For this review, take the finished solid that the model builds, in its own axes (mm). Face numbers are marked on the shaded views. Coordinates: 2 decimals unless noted, no trailing zeros. Write each loop counter-clockwise with the first axis right and the second up, starting at its lowest first coordinate (ties: lowest second). Pieces come first, ordered by that corner, then holes. Notation, with made-up numbers: M -20.5,14.25 L 18.5,14.25 A33 ccw 18.5,53.25 Z; hole C -2,-17 d2. An arc over 180 degrees is marked long. Return JSON: item names as keys, results as strings.
Autodesk Inventor part; units mm, degrees
ref_plane "YZ Plane" through (0, 0, 0) normal (1, 0, 0) x (0, 1, 0)
ref_plane "XZ Plane" through (0, 0, 0) normal (0, 1, 0) x (-1, 0, 0)
ref_plane "XY Plane" through (0, 0, 0) normal (0, 0, 1) x (1, 0, 0)
sketch "0" plane through (0, 0, 0) normal (0, 0, 1) x (1, 0, 0)
  line L0 (4, 55.5) -> (4, 61.5)
  line L1 (4, 61.5) -> (14, 61.5)
  line L2 (14, 61.5) -> (14, 55.5)
  line L3 (20, 55.5) -> (18.5, 55.5)
  line L4 (18.5, 55.5) -> (18.5, 49.25)
  line L5 (18.5, 40.5) -> (15.5, 40.5)
  line L6 (15.5, 40.5) -> (15.5, 46.75)
  line L7 (14.25, 49.25) -> (15.5, 49.25)
  line L8 (19.75, 49.25) -> (19.75, 46.75)
  line L9 (19.75, 46.75) -> (18.5, 46.75)
  line L10 (14.25, 46.75) -> (14.25, 49.25)
  line L11 (15.5, 49.25) -> (15.5, 55.5)
  line L12 (15.5, 46.75) -> (14.25, 46.75)
  line L13 (18.5, 49.25) -> (19.75, 49.25)
  line L14 (15.5, 55.5) -> (14, 55.5)
  line L15 (20, 61.5) -> (30, 61.5)
  line L16 (20, 55.5) -> (20, 61.5)
  line L17 (18.5, 46.75) -> (18.5, 40.5)
  line L18 (-30, 61.5) -> (-20, 61.5)
  line L19 (-20, 61.5) -> (-20, 55.5)
  line L20 (-14, 55.5) -> (-15.5, 55.5)
  line L21 (-15.5, 55.5) -> (-15.5, 49.25)
  line L22 (-15.5, 40.5) -> (-18.5, 40.5)
  line L23 (-18.5, 40.5) -> (-18.5, 46.75)
  line L24 (-19.75, 49.25) -> (-18.5, 49.25)
  line L25 (-14.25, 49.25) -> (-14.25, 46.75)
  line L26 (-14.25, 46.75) -> (-15.5, 46.75)
  line L27 (-19.75, 46.75) -> (-19.75, 49.25)
  line L28 (-18.5, 49.25) -> (-18.5, 55.5)
  line L29 (-18.5, 46.75) -> (-19.75, 46.75)
  line L30 (-15.5, 49.25) -> (-14.25, 49.25)
  line L31 (-18.5, 55.5) -> (-20, 55.5)
  line L32 (-14, 61.5) -> (-4, 61.5)
  line L33 (-14, 55.5) -> (-14, 61.5)
  line L34 (-4, 61.5) -> (-4, 55.5)
  line L35 (-15.5, 46.75) -> (-15.5, 40.5)
  line L36 (-3, 55.5) -> (-4, 55.5)
  line L37 (3, 55.5) -> (4, 55.5)
  line L38 (30, 61.5) -> (30, 55.5)
  circle A0 centre (0, 0) radius 18
  line L39 (30, 55.5) -> (30, -4)
  line L40 (-30, -4) -> (-30, 61.5)
  arc A1 (-30, -4) -> (30, -4) centre (0, 8.5) ccw
  line L41 (-3, 19.5) -> (-3, 29.5)
  line L42 (-3, 29.5) -> (3, 29.5)
  line L43 (3, 29.5) -> (3, 19.5)
  line L44 (3, 19.5) -> (-3, 19.5)
  line L45 (-3, 35.5) -> (-3, 45.5)
  line L46 (3, 45.5) -> (3, 35.5)
  line L47 (3, 35.5) -> (-3, 35.5)
  circle A2 centre (0, 32.5) radius 1.6
  line L48 (-3, 45.5) -> (3, 45.5)
  line L49 (-3, 55.5) -> (3, 55.5)
  point P0 (-30, -4)
  point P1 (30, -4)
sketch "Эскиз3" plane through (0, 0, 0) normal (0, 0, 1) x (1, 0, 0)
  circle A0 centre (0, 0) radius 18
  circle A1 centre (0, 32.5) radius 1.6
  line L0 (30, 55.5) -> (30, -4)
  line L1 (-30, -4) -> (-30, 61.5)
  line L2 (-30, 61.5) -> (-20, 61.5)
  line L3 (30, 61.5) -> (30, 55.5)
  line L4 (20, 61.5) -> (30, 61.5)
  line L5 (20, 55.5) -> (20, 61.5)
  line L6 (20, 55.5) -> (18.5, 55.5)
  line L7 (18.5, 55.5) -> (18.5, 49.25)
  line L8 (18.5, 49.25) -> (19.75, 49.25)
  line L9 (19.75, 49.25) -> (19.75, 46.75)
  line L10 (19.75, 46.75) -> (18.5, 46.75)
  line L11 (18.5, 46.75) -> (18.5, 40.5)
  line L12 (18.5, 40.5) -> (15.5, 40.5)
  line L13 (15.5, 40.5) -> (15.5, 46.75)
  line L14 (15.5, 46.75) -> (14.25, 46.75)
  line L15 (14.25, 46.75) -> (14.25, 49.25)
  line L16 (14.25, 49.25) -> (15.5, 49.25)
  line L17 (15.5, 49.25) -> (15.5, 55.5)
  line L18 (15.5, 55.5) -> (14, 55.5)
  line L19 (4, 61.5) -> (14, 61.5)
  line L20 (4, 55.5) -> (4, 61.5)
  line L21 (-3, 55.5) -> (3, 55.5)
  line L22 (3, 55.5) -> (4, 55.5)
  line L23 (14, 61.5) -> (14, 55.5)
  line L24 (-14, 61.5) -> (-4, 61.5)
  line L25 (-4, 61.5) -> (-4, 55.5)
  line L26 (-14, 55.5) -> (-15.5, 55.5)
  line L27 (-15.5, 55.5) -> (-15.5, 49.25)
  line L28 (-18.5, 49.25) -> (-18.5, 55.5)
  line L29 (-18.5, 55.5) -> (-20, 55.5)
  line L30 (-20, 61.5) -> (-20, 55.5)
  line L31 (-19.75, 49.25) -> (-18.5, 49.25)
  line L32 (-19.75, 46.75) -> (-19.75, 49.25)
  line L33 (-18.5, 46.75) -> (-19.75, 46.75)
  line L34 (-18.5, 40.5) -> (-18.5, 46.75)
  line L35 (-15.5, 40.5) -> (-18.5, 40.5)
  line L36 (-15.5, 46.75) -> (-15.5, 40.5)
  line L37 (-14.25, 46.75) -> (-15.5, 46.75)
  line L38 (-14.25, 49.25) -> (-14.25, 46.75)
  line L39 (-15.5, 49.25) -> (-14.25, 49.25)
  arc A2 (-30, -4) -> (30, -4) centre (0, 8.5) ccw
  line L40 (3, 29.5) -> (3, 19.5)
  line L41 (-3, 29.5) -> (3, 29.5)
  circle A3 centre (0, 0) radius 18
  circle A4 centre (0, 32.5) radius 1.6
  line L42 (-3, 45.5) -> (3, 45.5)
  line L43 (3, 45.5) -> (3, 35.5)
  line L44 (3, 35.5) -> (-3, 35.5)
  line L45 (-3, 35.5) -> (-3, 45.5)
  line L46 (-3, 29.5) -> (3, 29.5)
  line L47 (3, 29.5) -> (3, 19.5)
  line L48 (3, 19.5) -> (-3, 19.5)
  line L49 (-3, 19.5) -> (-3, 29.5)
  line L50 (18.5, 40.5) -> (15.5, 40.5)
  line L51 (15.5, 40.5) -> (15.5, 46.75)
  line L52 (18.5, 46.75) -> (18.5, 40.5)
  line L53 (19.75, 49.25) -> (19.75, 46.75)
  line L54 (14.25, 46.75) -> (14.25, 49.25)
  line L55 (18.5, 55.5) -> (18.5, 49.25)
  line L56 (15.5, 49.25) -> (15.5, 55.5)
  line L57 (20, 61.5) -> (20, 55.5)
  line L58 (14, 55.5) -> (14, 61.5)
  line L59 (4, 55.5) -> (-4, 55.5)
  line L60 (-4, 55.5) -> (-4, 61.5)
  line L61 (4, 61.5) -> (4, 55.5)
  line L62 (-20, 55.5) -> (-20, 61.5)
  line L63 (-14, 61.5) -> (-14, 55.5)
  line L64 (-15.5, 55.5) -> (-15.5, 49.25)
  line L65 (-18.5, 49.25) -> (-18.5, 55.5)
  line L66 (-14.25, 49.25) -> (-14.25, 46.75)
  line L67 (-19.75, 46.75) -> (-19.75, 49.25)
  line L68 (-15.5, 46.75) -> (-15.5, 40.5)
  line L69 (-15.5, 40.5) -> (-18.5, 40.5)
  line L70 (-18.5, 40.5) -> (-18.5, 46.75)
  line L71 (-14, 55.5) -> (-15.5, 55.5)
  line L72 (-18.5, 55.5) -> (-20, 55.5)
  line L73 (-19.75, 49.25) -> (-18.5, 49.25)
  line L74 (-15.5, 49.25) -> (-14.25, 49.25)
  line L75 (-14.25, 46.75) -> (-15.5, 46.75)
  line L76 (-18.5, 46.75) -> (-19.75, 46.75)
  line L77 (20, 55.5) -> (18.5, 55.5)
  line L78 (15.5, 55.5) -> (14, 55.5)
  line L79 (14.25, 49.25) -> (15.5, 49.25)
  line L80 (18.5, 49.25) -> (19.75, 49.25)
  line L81 (19.75, 46.75) -> (18.5, 46.75)
  line L82 (15.5, 46.75) -> (14.25, 46.75)
  line L83 (-30, 61.5) -> (-20, 61.5)
  line L84 (-14, 61.5) -> (-4, 61.5)
  line L85 (20, 61.5) -> (30, 61.5)
  line L86 (14, 61.5) -> (4, 61.5)
  line L87 (30, 61.5) -> (30, -4)
  line L88 (-30, -4) -> (-30, 61.5)
  arc A5 (-30, -4) -> (30, -4) centre (0, 8.5) ccw
  point P0 (0, 0)
extrude "Выдавливание2" add sketch "Эскиз3" along normal blind 10
properties part number "Крепление_мотора2_платформа"
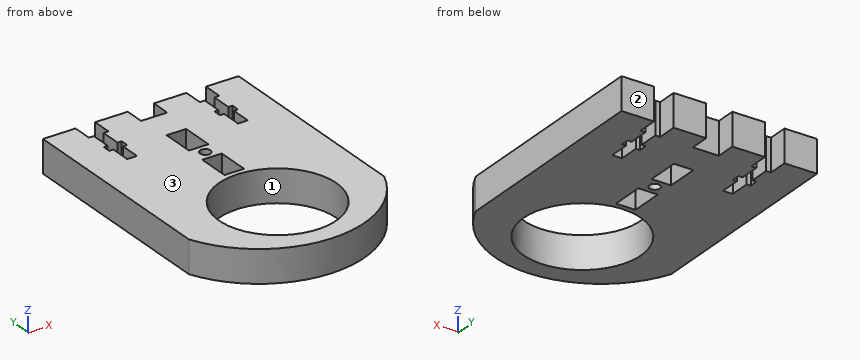
1. We need section A-A (x = 0). State the section outline as (y, z) points.
Checks:
{"outline": "M -24,0 L -18,0 L -18,10 L -24,10 Z; M 18,0 L 19.5,0 L 19.5,10 L 18,10 Z; M 29.5,0 L 30.9,0 L 30.9,10 L 29.5,10 Z; M 34.1,0 L 35.5,0 L 35.5,10 L 34.1,10 Z; M 45.5,0 L 55.5,0 L 55.5,10 L 45.5,10 Z"}
2. We need section D-D (x = -6.5). State the section outline as (y, z) points, plus the area to 3 significant figures.
Checks:
{"outline": "M -23.34,0 L -16.79,0 L -16.79,10 L -23.34,10 Z; M 16.79,0 L 61.5,0 L 61.5,10 L 16.79,10 Z", "area": "513 mm2"}
3. We need section C-C (y = 44.5). State the section outline as (x, z) points, plus the area to 3 significant figures.
Checks:
{"outline": "M -30,0 L -18.5,0 L -18.5,10 L -30,10 Z; M -15.5,0 L -3,0 L -3,10 L -15.5,10 Z; M 3,0 L 15.5,0 L 15.5,10 L 3,10 Z; M 18.5,0 L 30,0 L 30,10 L 18.5,10 Z", "area": "480 mm2"}
4. Wall thickness on L1, parallel to Y at x = 0, z = 3.5; L2, parallel to X at y = 23, z = 2; L3, parallel to X at y = 54.5, z = 7.5: over which ranges is each line inside the solid? List them lowest first. Write a range as from..to.
Checks:
{"L1": "-24..-18, 18..19.5, 29.5..30.9, 34.1..35.5, 45.5..55.5", "L2": "-30..-3, 3..30", "L3": "-30..-18.5, -15.5..15.5, 18.5..30"}
5. We need section B-B (y = 32.5). State the section outline as (x, z) points.
Checks:
{"outline": "M -30,0 L -1.6,0 L -1.6,10 L -30,10 Z; M 1.6,0 L 30,0 L 30,10 L 1.6,10 Z"}
6. Draft analysis for pull direction Y (two halves, no side actions). For the marked faces 1, 2 and 3, state which applies: +Y half, -Y half, draft (parallel to the pull), parting line (faces both ways), or undercut.
Checks:
{"face 1": "undercut", "face 2": "+Y half", "face 3": "draft"}
7. Clearance check with flat-ended pins moving along their axes: pin 1 Ø1.4 at (x, z) = (-15, 2.5) entering from -Y; pin 2 Ø1 at (x, z) = (15, 3.5) entering from -Y; pin 3 Ø5 at (x, z) = (-0.5, 6.5) entering from +Y. State where each tip first meets the part, or that it passes through.
Checks:
{"pin 1": "y = -20.68", "pin 2": "y = -20.59", "pin 3": "y = 55.5"}
